from build123d import *

# Parameters (mm, degrees)
SKETCH_1_W          = 75.027591161
SKETCH_1_H          = 49.216029974
EXTRUDE_1_DEPTH     = 11
CUT_EXTRUDE_START   = -11
SKETCH_2_R          = 1
SKETCH_2_R_2        = 1.5
SKETCH_2_R_3        = 0.8
CUT_EXTRUDE_1_DEPTH = 3
SKETCH_2_4_R        = 12.2
SKETCH_2_4_W        = 5
SKETCH_2_4_H        = 5
SKETCH_2_4_W_2      = 41.827591161
SKETCH_2_4_H_2      = 24
CUT_EXTRUDE_3_DEPTH = 80.722605558
SKETCH_4_W          = 88
SKETCH_4_H          = 55.1
SKETCH_4_R          = 2
SKETCH_4_W_2        = 50.6
SKETCH_4_H_2        = 24
EXTRUDE_2_DEPTH     = 1
SKETCH_5_R          = 2.5
CUT_EXTRUDE_4_DEPTH = 91.910079199
SKETCH_7_W          = 9.2
SKETCH_7_H          = 5
CUT_EXTRUDE_6_DEPTH = 2
SKETCH_8_R          = 1
SKETCH_8_R_2        = 0.5
CUT_EXTRUDE_7_DEPTH = 91.910079199
SKETCH_9_W          = 16
SKETCH_9_H          = 29.2
CUT_EXTRUDE_8_DEPTH = 2


with BuildPart() as part:
    # 草图1 → 凸台-拉伸1 (new body)
    with BuildSketch(Plane.XY):
        with Locations((-37.513795581, 0)):
            Rectangle(SKETCH_1_W, SKETCH_1_H)
    extrude(amount=EXTRUDE_1_DEPTH)

    # 草图2 → 切除-拉伸1 (cut)
    with BuildSketch(Plane(origin=(0, 0, 0), x_dir=(-1, 0, 0), z_dir=(0, 0, -1)).offset(CUT_EXTRUDE_START)):
        with Locations(Location((11.3, 14.7, 0), (0, 0, 180))):
            Circle(SKETCH_2_R)
        with Locations(Location((11.3, -14.7, 0), (0, 0, 180))):
            Circle(SKETCH_2_R)
        with Locations(Location((26.7, 3.6, 0), (0, 0, 180))):
            Circle(SKETCH_2_R_2)
        with Locations(Location((49.1, 15.4, 0), (0, 0, 180))):
            Circle(SKETCH_2_R_3)
        with Locations(Location((49.1, -15.4, 0), (0, 0, 180))):
            Circle(SKETCH_2_R_3)
    extrude(amount=CUT_EXTRUDE_1_DEPTH, mode=Mode.SUBTRACT)

    # 草图2<4> → 切除-拉伸3 (cut, through all)
    with BuildSketch(Plane(origin=(0, 0, 0), x_dir=(-1, 0, 0), z_dir=(0, 0, -1))):
        with Locations((13.2, 0)):
            Circle(SKETCH_2_4_R)
        with Locations((2.5, 22.108014987)):
            Rectangle(SKETCH_2_4_W, SKETCH_2_4_H)
        with Locations((2.5, -22.108014987)):
            Rectangle(SKETCH_2_4_W, SKETCH_2_4_H)
        with Locations((54.113795581, 0)):
            Rectangle(SKETCH_2_4_W_2, SKETCH_2_4_H_2)
    extrude(amount=-CUT_EXTRUDE_3_DEPTH, mode=Mode.SUBTRACT)

    # 草图4 → 凸台-拉伸2 (add)
    with BuildSketch(Plane(origin=(0, 0, 0), x_dir=(-1, 0, 0), z_dir=(0, 0, -1))):
        with Locations((41.8, 0)):
            Rectangle(SKETCH_4_W, SKETCH_4_H)
        with Locations((0.8, 24.55)):
            Circle(SKETCH_4_R, mode=Mode.SUBTRACT)
        with Locations((0.8, -24.55)):
            Circle(SKETCH_4_R, mode=Mode.SUBTRACT)
        with Locations((82.8, -24.55)):
            Circle(SKETCH_4_R, mode=Mode.SUBTRACT)
        with Locations((82.8, 24.55)):
            Circle(SKETCH_4_R, mode=Mode.SUBTRACT)
        with Locations((58.5, 0)):
            Rectangle(SKETCH_4_W_2, SKETCH_4_H_2, mode=Mode.SUBTRACT)
    extrude(amount=EXTRUDE_2_DEPTH)

    # 草图5 → 切除-拉伸4 (cut, through all)
    with BuildSketch(Plane.XY.offset(11)):
        with Locations((-21.82670273, 8.62670273)):
            Circle(SKETCH_5_R)
    extrude(amount=-CUT_EXTRUDE_4_DEPTH, mode=Mode.SUBTRACT)

    # 草图7 → 切除-拉伸6 (cut)
    with BuildSketch(Plane(origin=(0, 0, -1), x_dir=(-1, 0, 0), z_dir=(0, 0, -1))):
        with Locations((22.2, -17.25)):
            Rectangle(SKETCH_7_W, SKETCH_7_H)
    extrude(amount=-CUT_EXTRUDE_6_DEPTH, mode=Mode.SUBTRACT)

    # 草图8 → 切除-拉伸7 (cut, through all)
    with BuildSketch(Plane.XY.offset(11)):
        with Locations((-26.4, -17.25)):
            Circle(SKETCH_8_R)
        with Locations((-24.2, -17.25)):
            Circle(SKETCH_8_R_2)
        with Locations((-22.2, -17.25)):
            Circle(SKETCH_8_R_2)
        with Locations((-20.2, -17.25)):
            Circle(SKETCH_8_R_2)
        with Locations((-18, -17.25)):
            Circle(SKETCH_8_R)
    extrude(amount=-CUT_EXTRUDE_7_DEPTH, mode=Mode.SUBTRACT)

    # 草图9 → 切除-拉伸8 (cut)
    with BuildSketch(Plane.XY.offset(11)):
        with Locations((-25.2, -2.6)):
            Rectangle(SKETCH_9_W, SKETCH_9_H)
    extrude(amount=-CUT_EXTRUDE_8_DEPTH, mode=Mode.SUBTRACT)


solid = part.part
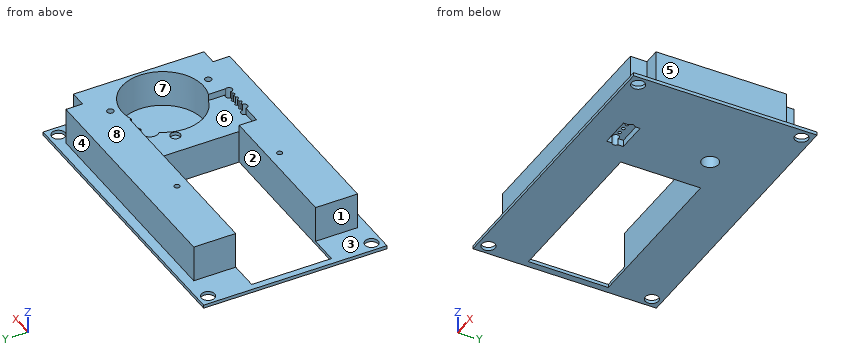
Source: CAD feature listing. Evaluate the final solid. Frame: model axes, mm. Face numbers are marked on the shaded views. A direction names the side the tool comes from. Give positions to 0.01 mm unless a question says otherwise; leave off trailing zeros. Write each loop counter-clockwise with the first axis right and the second up, starting at its lowest first coordinate (ties: lowest second). Pieces come first, ordered by that corner, then holes. Notation, with made-up numbers: M -23,74.25 L -3,74.25 A11 cw -3,81.25 Z; hole C 83,1 d5. An arc over 180 degrees is marked long. Return JSON: item names as keys, results as strings. Group by question number.
1) Cut plane C-C, the plane z = 10. Give the number of separate pieces and of enclosed holes in the cut face, then the cut area to 3 significant figures.
2) Cut plane D-D, the plane x = -79.5. Output: boundary loops of the cut face in (y, z), then the cut area to 3 significant figures.
3) Cut plane B-B, the plane y = -7.5. Output: boundary loops of the cut face in (x, z), then the cut area to 3 significant figures.
4) Draft query along X for the marked faces 5, 6, 7 and 8. Return one class per face: released by +X, released by -X, zero draft, split by the parting line, or undercut.
5) Set-up query: the marked faces 1, 2, 3 and 4. Return all of +Z, -Z, +X, -X, +Y, -Y with unobstructed straight access to the full face (end or side cutting, diameter ignored); none if empty.
6) Cut plane A-A, the plane x = -57. Output: boundary loops of the cut face in (y, z).
7) First-contact query: pin 1 Ø6 at (x, y) = (-21.83, 8.63) entering from +Z; pin 2 Ø3.5 at (x, z) = (-38, 2.5) entering from -Y; pin 3 Ø1.4 at (x, y) = (-49.1, -15.4) entering from +Z; pin 4 Ø3.5 at (x, y) = (-0.8, -24.55) entering from -Z. Flat tips, straight axial feed; report the tip coordinate or a pass-through.
8) Ray query, L1, parallel to X at y = -17.25, z = 6; L2, parallel to Y at x = -23.5, z = 6; L3, parallel to Y at x = -53.5, z = 3.5. Return the intervals inside material, ascending.
Data:
{
 "1": {"separate pieces": "1", "enclosed holes": "4", "area": "1,830 mm²"},
 "2": {"outline": "M -27.55,-1 L -12,-1 L -12,0 L -27.55,0 Z; M 12,-1 L 27.55,-1 L 27.55,0 L 12,0 Z", "area": "31.1 mm²"},
 "3": {"outline": "M -85.8,-1 L -83.8,-1 L -83.8,0 L -85.8,0 Z; M -33.2,-1 L 2.2,-1 L 2.2,0 L 0,0 L 0,11 L -3.58,11 L -3.58,0 L -22.82,0 L -22.82,9 L -33.2,9 Z", "area": "170 mm²"},
 "4": {"face 5": "released by +X", "face 6": "undercut", "face 7": "undercut", "face 8": "zero draft"},
 "5": {"face 1": "+Z, -X, +Y, -Y", "face 2": "+Z, -Z", "face 3": "+Z", "face 4": "+Z, +X, -X, +Y"},
 "6": {"outline": "M -27.55,-1 L -12,-1 L -12,11 L -24.61,11 L -24.61,0 L -27.55,0 Z; M 12,-1 L 27.55,-1 L 27.55,0 L 24.61,0 L 24.61,11 L 12,11 Z"},
 "7": {"pin 1": "stops at z = 9", "pin 2": "stops at y = -24.61", "pin 3": "stops at z = 8", "pin 4": "passes through"},
 "8": {"L1": "x = -75.03 to -27.4, -25.4 to -24.7, -23.7 to -22.7, -21.7 to -20.7, -19.7 to -19, -17 to 0", "L2": "y = -24.61 to -6.54, 6.54 to 6.77, 10.48 to 24.61", "L3": "y = -24.61 to -12, 12 to 24.61"}
}
